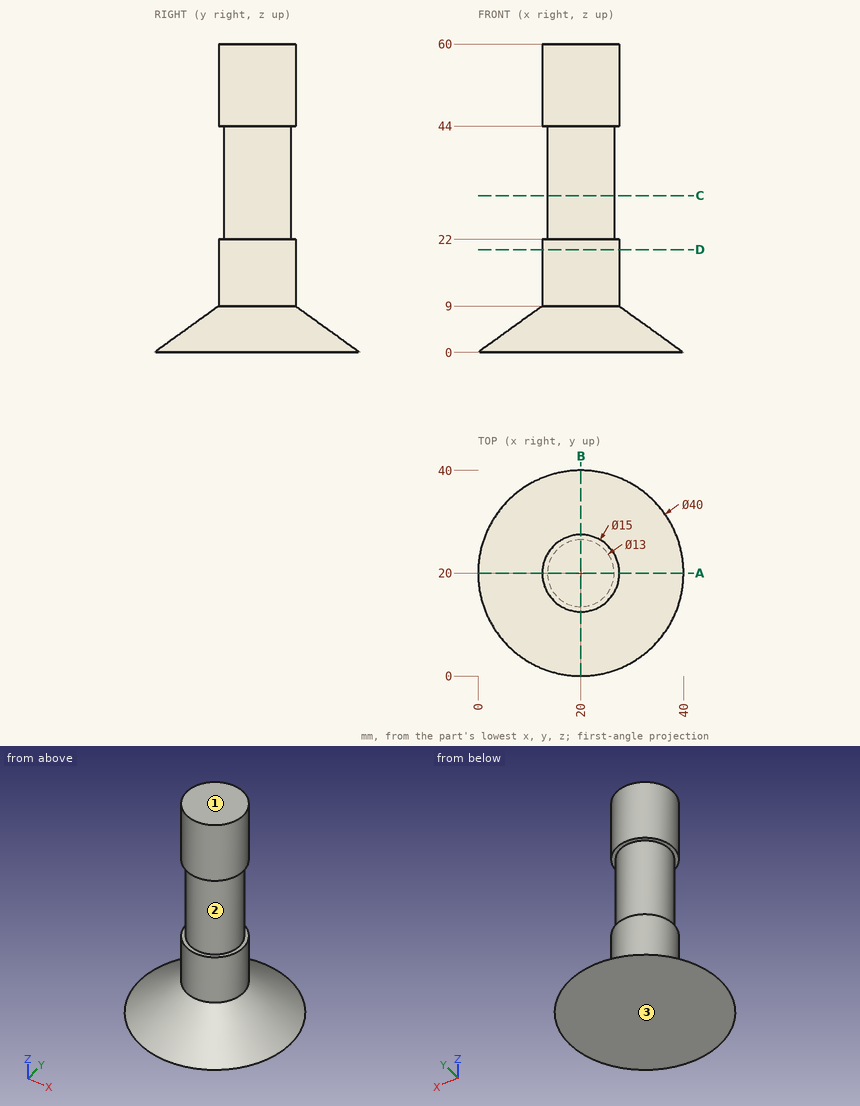
Design review of the part shown in the three views and the two pictorial views. Dimensions are in mm from the part's minimum x, y and z. Give positions to 0.01 mm unless a question says otherwise; leave off trailing zeros. Loops run counter-clockwise (first coordinate to the right, second up) from the corner with the lowest first, then second, coordinate; pieces in that order, holes last. Notation, with made-up numbers: (36, 40) - (84, 40) arc R26 cw to (84, 68) - close; hole circle Ø4 at (50, 4.25). An arc over 180 degrees is marked (long way). Use CSV: the item, a comma, the result in double quotes. Start each with the question number.
1. Add section A-A (y = 20). State the section outline as (x, z) points.
2. Wall thickness on L1, parallel to Y at x = 20, z = 31; L2, parallel to X at y = 26, z = 28; L3, parallel to X at y = 20.5, z = 8.5: over which ranges is each line inside the solid? List them lowest first.
3. Add section D-D (z = 20). State the section outline as (x, y) points.
4. Insertion check: P1, Ø4, axis at y = 13, z = 28, coming from the -X side; P2, Ø12, axis at x = 14, z = 50.5, coming from the +Y side; P3, Ø12, axis at x = 12.5, z = 35.5, coming from the +Y side. Each pin has a flat end and moves straight along its axis. Give the tip position at first contact, or say it passes through.
5. Draft analysis for pull direction Z (two halves, no side actions). For the marked faces 1, 2 and 3, state which applies: released by +Z, released by -Z, zero draft, split by the parting line, or undercut.
6. Add section C-C (z = 30.5). State the section outline as (x, y) points.
Results found:
1,outline,"(0, 0) - (40, 0) - (27.5, 9) - (27.5, 22) - (26.5, 22) - (26.5, 44) - (27.5, 44) - (27.5, 60) - (12.5, 60) - (12.5, 44) - (13.5, 44) - (13.5, 22) - (12.5, 22) - (12.5, 9) - close"
2,L1,"y = 13.5 to 26.5"
2,L2,"x = 17.5 to 22.5"
2,L3,"x = 11.82 to 28.18"
3,outline,"circle Ø15 at (20, 20)"
4,P1,"stops at x = 15.85"
4,P2,"stops at y = 27.5"
4,P3,"stops at y = 26.32"
5,face 1,"released by +Z"
5,face 2,"undercut"
5,face 3,"released by -Z"
6,outline,"circle Ø13 at (20, 20)"
